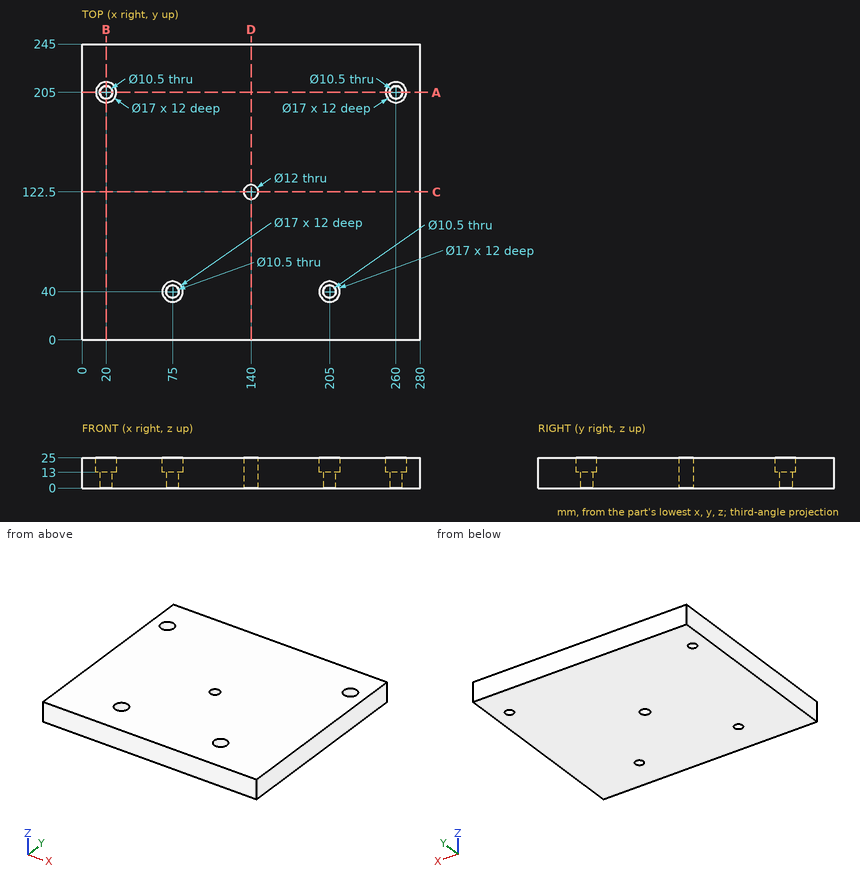
Could you check a few things on this drawing? It's one solid part, dimensions in mm from its lowest x, y, z. Round coordinates to 2 decimals unless told otherwise and drop trailing zeros. Loops run counter-clockwise (first coordinate to the right, second up) from the corner with the lowest first, then second, coordinate; pieces in that order, holes last.
Q1. For P1, Ø8.5, axis at x = 71, y = 40.5, coming from the +Z side; P2, Ø2, axis at x = 123, z = 17.5, coming from the -Y side; P3, Ø9.5, axis at x = 140, y = 122.5, coming from the -Z side, each with a flat end and sliding along its axis, tell me the tip position at first contact or that it passes through.
Q2. I want a section at A-A (y = 205). Write out the boundary of the cut face in (x, z).
Q3. I want a section at B-B (x = 20). Write out the boundary of the cut face in (y, z).
Q4. Please list where these lines run through material, in increasing order: L1, parallel to Y at x = 75, z = 3.25; L2, parallel to Y at x = 205, z = 20.5; L3, parallel to X at y = 126, z = 19.5.
Q5. I want a section at D-D (x = 140). Write out the boundary of the cut face in (y, z), and give its area (4 significant figures).
Q6. I want a section at C-C (y = 122.5). Write out the boundary of the cut face in (x, z), and give its area (3 significant figures).
Answer below:
1. P1: stops at z = 13
1. P2: stops at y = 0
1. P3: passes through
2. outline: (0, 0) - (14.75, 0) - (14.75, 13) - (11.5, 13) - (11.5, 25) - (0, 25) - close; (25.25, 0) - (254.75, 0) - (254.75, 13) - (251.5, 13) - (251.5, 25) - (28.5, 25) - (28.5, 13) - (25.25, 13) - close; (265.25, 0) - (280, 0) - (280, 25) - (268.5, 25) - (268.5, 13) - (265.25, 13) - close
3. outline: (0, 0) - (199.75, 0) - (199.75, 13) - (196.5, 13) - (196.5, 25) - (0, 25) - close; (210.25, 0) - (245, 0) - (245, 25) - (213.5, 25) - (213.5, 13) - (210.25, 13) - close
4. L1: y = 0 to 34.75, 45.25 to 245
4. L2: y = 0 to 31.5, 48.5 to 245
4. L3: x = 0 to 135.13, 144.87 to 280
5. outline: (0, 0) - (116.5, 0) - (116.5, 25) - (0, 25) - close; (128.5, 0) - (245, 0) - (245, 25) - (128.5, 25) - close
5. area: 5,825 mm2
6. outline: (0, 0) - (134, 0) - (134, 25) - (0, 25) - close; (146, 0) - (280, 0) - (280, 25) - (146, 25) - close
6. area: 6,700 mm2
